from build123d import *

# Parameters (mm, degrees)
BOSS_EXTRUDE1_DEPTH      = 3.175
SKETCH2_R                = 6.477
SKETCH2_R_2              = 1.27
CUT_EXTRUDE1_DEPTH       = 252.527339468
Q_0_332_DIAMETER_HOLE1_D = 8.4328
FILLET1_R                = 12.7


with BuildPart() as part:
    # Sketch1 → Boss-Extrude1 (new, symmetric)
    with BuildSketch(Plane(origin=(0, 0, 0), x_dir=(1, 0, 0), z_dir=(0, 1, 0))):
        with BuildLine():
            Line((0, 177.8), (0, 0))
            Line((0, 0), (177.8, 0))
            ThreePointArc((177.8, 0), (125.723585695, 125.723585695), (0, 177.8))
        make_face()
    extrude(amount=BOSS_EXTRUDE1_DEPTH, both=True)

    # Sketch2 → Cut-Extrude1 (cut, through all)
    with BuildSketch(Plane(origin=(0, 3.175, 0), x_dir=(1, 0, 0), z_dir=(0, 1, 0))):
        with Locations(Location((101.6, 101.6, 0), (0, 0, 270))):
            Circle(SKETCH2_R)
        with Locations(Location((101.6, 91.2749, 0), (0, 0, 270))):
            Circle(SKETCH2_R_2)
        with Locations(Location((101.6, 111.9251, 0), (0, 0, 270))):
            Circle(SKETCH2_R_2)
    extrude(amount=-CUT_EXTRUDE1_DEPTH, mode=Mode.SUBTRACT)

    # Q (0.332) Diameter Hole1 (through all)
    with Locations(Plane(origin=(0, 3.175, 0), x_dir=(1, 0, 0), z_dir=(0, 1, 0))):
        with Locations((19.05, 152.4), (152.4, 19.05)):
            Hole(Q_0_332_DIAMETER_HOLE1_D / 2)

    # Fillet1
    fillet1_edges = [part.edges().sort_by_distance(p)[0] for p in [
        (0, 0, 0),
        (0, 0, -177.8),
        (177.8, 0, 0),
    ]]
    fillet(fillet1_edges, radius=FILLET1_R)


solid = part.part
Part model, mm, in its own coordinate system. Coordinates: 2 decimals unless noted, no trailing zeros. Loops run counter-clockwise (first coordinate to the right, second up) from the corner with the lowest first, then second, coordinate; pieces in that order, holes last. Notation, with made-up numbers: M -27,-3.5 L 17,-3.5 A25 ccw 17,16.5 Z; hole C 24,71.25 d3. An arc over 180 degrees is marked long. Use a Markdown table: item, result. Add a question column.
Q1. Probe L1, parallel to Z at x = 99, y = 3; L2, parallel to X at y = 0, z = -152.4; L3, parallel to Z at x = 19.05, y = -0.75. List the from-to ranges inside material, lowest first.
Q2. Cut at C-C (x = 152.4). Write the cut outline in (y, z) (3 decimals).
Q3. Mould opens along Z. For faces 1 (the cylindrical face through (3.62, 0.04, -3.82)), 2 (the flat face through (68, 3.175, -70)), 3 (the cylindrical face through (126.964, 0.044, -124.471)), 4 (the cylindrical face through (95.854, 0.044, -98.611)) say: +Z half, -Z half, draft (parallel to the pull), parting line (faces both ways), or undercut.
Q4. Cut at A-A (y = 1). Write the cut outline in (x, z).
Q5. Pin check, flat tips, straight feed: P1, Ø3, axis at y = 1, z = -135, coming from the +X side; P2, Ø1, axis at x = 118, y = -1, coming from the -Z side; P3, Ø1.5, axis at y = 2.5, z = -24.5, coming from the +X side. Stop position of each tip, or through.
Q6. Cut at D-D (x = 80.5). Write the cut outline in (y, z) (3 decimals).
Q7. Cut at B-B (z = -101.6). Write the cut outline in (x, y) (3 decimals), and give its area (3 significant figures).
Worked out:
| question | item | result |
|---|---|---|
| 1 | L1 | z = -147.69 to -107.53, -95.67 to 0 |
| 1 | L2 | x = 0 to 14.83, 23.27 to 91.58 |
| 1 | L3 | z = -176.78 to -156.62, -148.18 to 0 |
| 2 | outline | M -3.175,-91.581 L 3.175,-91.581 L 3.175,-23.266 L -3.175,-23.266 Z; M -3.175,-14.834 L 3.175,-14.834 L 3.175,0 L -3.175,0 Z |
| 3 | face 1 | +Z half |
| 3 | face 2 | draft |
| 3 | face 3 | -Z half |
| 3 | face 4 | undercut |
| 4 | outline | M 0,-164.61 A12.7 ccw 13.68,-177.27 A177.8 ccw 177.27,-13.68 A12.7 ccw 164.61,0 L 12.7,0 A12.7 ccw 0,-12.7 Z; hole C 19.05,-152.4 d8.43; hole C 101.6,-101.6 d12.95; hole C 101.6,-111.93 d2.54; hole C 101.6,-91.27 d2.54; hole C 152.4,-19.05 d8.43 |
| 5 | P1 | stops at x = 117.43 |
| 5 | P2 | stops at z = -133.44 |
| 5 | P3 | stops at x = 176.21 |
| 6 | outline | M -3.175,-158.533 L 3.175,-158.533 L 3.175,0 L -3.175,0 Z |
| 7 | outline | M 0,-3.175 L 95.123,-3.175 L 95.123,3.175 L 0,3.175 Z; M 108.077,-3.175 L 145.912,-3.175 L 145.912,3.175 L 108.077,3.175 Z |
| 7 | area | 844 mm2 |
